For this review, take the finished solid that the model builds, in its own axes (mm). A direction names the side the tool comes from. Coordinates: 2 decimals unless noted, no trailing zeros. Loops run counter-clockwise (first coordinate to the right, second up) from the corner with the lowest first, then second, coordinate; pieces in that order, holes last.
1. Machinability: for faces 1 (the face through (32, 13, 3)), 2 (the face through (40, 1, 10)), 3 (the face through (31.077, 16.54, 18.521)), 4 (the face through (34, -2, 10)), which of the approach directions +Z, -Z, +X, -X, +Y, -Y give a long, thin tool a straight path to every point of the face, cutting with its end or side? Answer none if there is none.
2. Take a section at D-D, the plane y = -16.5. State the section outline as (x, z) points.
3. To check wall thickness, follow probe 1 along Y at (x, z) = (5.75, 3.55); probe 2 along Z at (x, y) = (5, 22.5); probe 3 along Z at (x, y) = (8, 32). State the ranges of each line that lie inside material, in increasing order.
4. Mouldability with a two-part tool opening along X and no side actions: class faces 5 (the face through (37.423, 12.807, 18.521)), 6 (the face through (0, 11, 10)), 7 (the face through (2.58, 32.93, 18.52)), 8 (the face through (20, 16, 15)) as pulls with the +X half, pulls with the -X half, needs draft (parallel to the pull), parting line crosses it, or undercut.
5. Take a section at A-A, the plane z = 10. State the section outline as (x, y) points, then the cut area to 3 significant figures.
6. Take a section at B-B, the plane x = 35. State the section outline as (y, z) points.
7. Take a section at C-C, the plane x = 17. State the section outline as (y, z) points, then the cut area to 3 significant figures.
8. Clearance check with flat-ended pins moving along their axes: P1, Ø3.5, axis at x = 34.25, y = 14.67, coming from the -Z side; P2, Ø0.9, axis at x = 6.5, z = 19, coming from the +Y side; P3, Ø2.5, axis at x = 33.5, z = 2, coming from the +Y side; P4, Ø5.5, axis at x = 5.75, y = 31.061, coming from the +Z side. State where each tip first meets the part, or that it passes through.
Solid Edge part; units mm, degrees
sketch "Sketch1" plane through (0, 0, 0) normal (0, 0, 1) x (1, 0, 0)
  line L0 (37.1162, 19.6582) -> (8.6162, 36.0457)
  line L1 (0, -2) -> (0, 31.061)
  line L2 (0, -2) -> (40, -2)
  line L3 (40, -2) -> (40, 14.6735)
  arc A0 (8.6162, 36.0457) -> (0, 31.061) centre (5.75, 31.061) ccw
  arc A1 (37.1162, 19.6582) -> (40, 14.6735) centre (34.25, 14.6735) cw
  circle A2 centre (34.25, 14.6735) radius 2.05
  circle A3 centre (5.75, 31.061) radius 2.05
extrude "Protrusion1" add sketch "Sketch1" along normal blind 20
sketch "Sketch2" plane through (20, 18.4055, 0) normal (0, 0, -1) x (1, 0, 0)
  line L0 (-12.125, -8.9749) -> (-16.375, -8.9749)
  line L1 (-16.375, -8.9749) -> (-18.5, -12.6555)
  line L2 (-18.5, -12.6555) -> (-16.375, -16.3361)
  line L3 (-16.375, -16.3361) -> (-12.125, -16.3361)
  line L4 (-12.125, -16.3361) -> (-10, -12.6555)
  line L5 (-10, -12.6555) -> (-12.125, -8.9749)
  line L6 (12.125, 7.4126) -> (10, 3.732)
  line L7 (10, 3.732) -> (12.125, 0.0514)
  line L8 (12.125, 0.0514) -> (16.375, 0.0514)
  line L9 (16.375, 0.0514) -> (18.5, 3.732)
  line L10 (18.5, 3.732) -> (16.375, 7.4126)
  line L11 (16.375, 7.4126) -> (12.125, 7.4126)
extrude "ExtrudedCutout_1" cut sketch "Sketch2" against normal blind 3
sketch "Sketch3" plane through (20, 17.4055, 20) normal (0, 0, 1) x (1, 0, 0)
  line L0 (-10, 13.6555) -> (-12.125, 17.3361)
  line L1 (-12.125, 17.3361) -> (-16.375, 17.3361)
  line L2 (-16.375, 17.3361) -> (-18.5, 13.6555)
  line L3 (-18.5, 13.6555) -> (-16.375, 9.9749)
  line L4 (-16.375, 9.9749) -> (-12.125, 9.9749)
  line L5 (-12.125, 9.9749) -> (-10, 13.6555)
  line L6 (18.5, -2.732) -> (16.375, 0.9486)
  line L7 (16.375, 0.9486) -> (12.125, 0.9486)
  line L8 (12.125, 0.9486) -> (10, -2.732)
  line L9 (10, -2.732) -> (12.125, -6.4126)
  line L10 (12.125, -6.4126) -> (16.375, -6.4126)
  line L11 (16.375, -6.4126) -> (18.5, -2.732)
extrude "ExtrudedCutout_2" cut sketch "Sketch3" against normal blind 3
sketch "Sketch4" plane through (40, 6.3367, 10) normal (1, 0, 0) x (0, 0, -1)
  line L0 (-5, -4.3367) -> (5, -4.3367)
  line L1 (5, -4.3367) -> (5, 30.4742)
  line L2 (5, 30.4742) -> (-5, 30.4742)
  line L3 (-5, 30.4742) -> (-5, -4.3367)
extrude "ExtrudedCutout_3" cut sketch "Sketch4" against normal blind 40
sketch "Sketch5" plane through (20, -2, 10) normal (0, -1, 0) x (0, 0, -1)
  circle A0 centre (0, 0) radius 4.5
extrude "ExtrudedCutout_4" cut sketch "Sketch5" against normal blind 4
sketch "Sketch6" plane through (20, -2, 10) normal (0, -1, 0) x (0, 0, -1)
  circle A0 centre (0, 0) radius 10
  circle A1 centre (0, 0) radius 4.5
extrude "ExtrudedProtrusion_2" add sketch "Sketch6" along normal blind 30
sketch "Sketch7" plane through (20, 2, 10) normal (0, 1, 0) x (1, 0, 0)
  line L0 (-20, -5) -> (-16, -5)
  line L1 (-16, -5) -> (-16, 5)
  line L2 (-16, 5) -> (-20, 5)
  line L3 (-20, 5) -> (-20, -5)
extrude "ExtrudedProtrusion_3" add sketch "Sketch7" along normal blind 15
Results list:
1. face 1: -Z
1. face 2: +Z, -Z, +X, +Y, -Y
1. face 3: +Z
1. face 4: +X, -Y
2. outline: circle Ø20 at (20, 10); hole circle Ø9 at (20, 10)
3. probe 1: y = -2 to 29.01, 33.11 to 36.81
3. probe 2: z = 0 to 5, 15 to 20
3. probe 3: z = 3 to 5, 15 to 17
4. face 5: undercut
4. face 6: pulls with the -X half
4. face 7: undercut
4. face 8: needs draft
5. outline: (0, -2) - (10, -2) - (10, -32) - (15.5, -32) - (15.5, 2) - (4, 2) - (4, 17) - (0, 17) - close; (24.5, -32) - (30, -32) - (30, -2) - (40, -2) - (40, 2) - (24.5, 2) - close
5. area: 514 mm2
6. outline: (-2, 0) - (10.99, 0) - (10.99, 3) - (12.77, 3) - (12.77, 5) - (2, 5) - (2, 15) - (12.77, 15) - (12.77, 17) - (10.99, 17) - (10.99, 20) - (-2, 20) - close; (16.58, 3) - (18.35, 3) - (18.35, 0) - (20.88, 0) - (20.88, 5) - (16.58, 5) - close; (16.58, 15) - (20.88, 15) - (20.88, 20) - (18.35, 20) - (18.35, 17) - (16.58, 17) - close
7. outline: (-32, 0.46) - (-2, 0.46) - (-2, 0) - (31.23, 0) - (31.23, 5) - (2, 5) - (2, 6.65) - (-32, 6.65) - close; (-32, 13.35) - (2, 13.35) - (2, 15) - (31.23, 15) - (31.23, 20) - (-2, 20) - (-2, 19.54) - (-32, 19.54) - close
7. area: 717 mm2
8. P1: passes through
8. P2: stops at y = 36.8
8. P3: stops at y = 22.46
8. P4: stops at z = 17
